Source: CAD feature listing. Evaluate the final solid. Frame: model axes, mm. A direction names the side the tool comes from. Coordinates: 2 decimals unless noted, no trailing zeros. Write each loop counter-clockwise with the first axis right and the second up, starting at its lowest first coordinate (ties: lowest second). Pieces come first, ordered by that corner, then holes. Notation, with made-up numbers: M 84.5,-0.75 L 127.5,-0.75 A19 ccw 127.5,23.25 Z; hole C 70,24 d10. An arc over 180 degrees is marked long. One line per item, written item: value. Start each with the question number.
Item 1: Set-up query: faces 1 (the flat face through (1, -7, -1.2)), 2 (the flat face through (-1, -7, 0)). Return all of +Z, -Z, +X, -X, +Y, -Y with unobstructed straight access to the full face (end or side cutting, diameter ignored); none if empty.
Item 2: Cut plane A-A, the plane y = -3. Output: boundary loops of the cut face in (x, z), then the cut area to 3 significant figures.
Item 3: Pin query (flat end, axial travel): P1, Ø1, axis at x = 25.5, y = -13, coming from the +Z side; P2, Ø1.3, axis at y = -4.5, z = -1, coming from the -X side; P3, Ø1, axis at y = -7, z = -1, coming from the +X side; P4, Ø3, axis at x = -39, z = -13, coming from the -Y side. Return the tip coordinate at first contact, or that it passes through.
Item 4: Cut plane C-C, the plane z = -17. Output: boundary loops of the cut face in (x, y), then the cut area to 3 significant figures.
Item 5: Cut plane B-B, the plane x = 57. Output: boundary loops of the cut face in (y, z).
Item 6: Ray query, L1, parallel to Y at x = -39.5, z = -15.5; L2, parallel to Z at x = -14, y = -5.5. Return the intervals inside material, ascending. Write a range as from..to.
```python
from build123d import *

# Parameters (mm, degrees)
F0_W     = 117.3113062978
F0_H     = 14.8764327168
F1_DEPTH = 1.2
F2_R     = 1
F4_DEPTH = 1.2


with BuildPart() as f1:
    # F0 (on Top) → F1 (new body)
    with BuildSketch(Plane.XY):
        with Locations((2.1252036095, -7.4382163584)):
            Rectangle(F0_W, F0_H)
    extrude(amount=-F1_DEPTH)

    # F2
    f2_edges = [f1.edges().sort_by_distance(p)[0] for p in [
        (-56.53045, -14.876433, -0.6),
        (60.780857, -14.876433, -0.6),
    ]]
    fillet(f2_edges, radius=F2_R)

    # F3 (on face) → F4 (join)
    with BuildSketch(Plane(origin=(0, 0, 0), x_dir=(-1, 0, 0), z_dir=(0, 1, 0))):
        Polygon((-60.7808567584, -1.2), (-60.7808567584, 0), (-100, 0), (-100, -18.8519991934), (100, -18.8519991934), (100, 0), (56.5304495394, 0), (56.5304495394, -1.2), align=None)
        Polygon((56.5304495394, 0), (0, 0), (-60.7808567584, 0), (-60.7808567584, -1.2), (56.5304495394, -1.2), align=None)
    extrude(amount=F4_DEPTH)


solid = f1.part
```
From the geometry:
1. face 1: -Z, +X, -X, -Y
1. face 2: +Z, +X, -X, +Y, -Y
2. outline: M -56.53,-1.2 L 60.78,-1.2 L 60.78,0 L -56.53,0 Z
2. area: 141 mm²
3. P1: stops at z = 0
3. P2: stops at x = -56.53
3. P3: stops at x = 60.78
3. P4: stops at y = 0
4. outline: M -100,0 L 100,0 L 100,1.2 L -100,1.2 Z
4. area: 240 mm²
5. outline: M -14.88,-1.2 L 0,-1.2 L 0,-18.85 L 1.2,-18.85 L 1.2,0 L -14.88,0 Z
6. L1: y = 0..1.2
6. L2: z = -1.2..0
